Can you work these out from the model? Positions are in its coordinate system, mm. A direction names the side the tool comes from. Round coordinates to 2 decimals unless told otherwise and drop trailing zeros. Loops run counter-clockwise (first coordinate to the right, second up) from the corner with the lowest first, then second, coordinate; pieces in that order, holes last.
from build123d import *

# Parameters (mm, degrees)
CUT_EXTRUDE1_START = 12.7
SKETCH2_R          = 12.7
CUT_EXTRUDE1_DEPTH = 76.2
FILLET2_R          = 15.24


with BuildPart() as part:
    # Sketch1 → Revolve1 (revolve)
    with BuildSketch(Plane.XY, mode=Mode.PRIVATE) as revolve1_sk:
        Polygon((0, 0), (0, 25.4), (50.8, 25.4), (50.8, 152.4), (101.6, 152.4), (101.6, 0), align=None)
    revolve(revolve1_sk.sketch.rotate(Axis((0, 0, 0), (0, 1, 0)), 270), axis=Axis((0, 0, 0), (0, 1, 0)))

    # Sketch2 → Cut-Extrude1 (cut)
    with BuildSketch(Plane.XZ.offset(CUT_EXTRUDE1_START)):
        with Locations(Location((-76.2, 0, 0), (0, 0, 270))):
            Circle(SKETCH2_R)
        with Locations(Location((76.2, 0, 0), (0, 0, 270))):
            Circle(SKETCH2_R)
    extrude(amount=-CUT_EXTRUDE1_DEPTH, mode=Mode.SUBTRACT)

    # Fillet2
    # the kernel refuses this fillet: 15.24 mm, written as the material it takes off along each edge
    with BuildSketch(Plane(origin=(0, 0, 0), x_dir=(0, 0, 1), z_dir=(-1, 0, 0))) as fillet2_piece_1:
        with BuildLine():
            CenterArc((101.6 - FILLET2_R, FILLET2_R), FILLET2_R, 270, 90)
            Line((101.6 - FILLET2_R, 0), (101.6, 0))
            Line((101.6, 0), (101.6, FILLET2_R))
        make_face()
    revolve(axis=Axis((0, 0, 0), (0, 1, 0)), mode=Mode.SUBTRACT)
    with BuildSketch(Plane(origin=(0, 152.4, 0), x_dir=(0, 0, 1), z_dir=(-1, 0, 0))) as fillet2_piece_2:
        with BuildLine():
            CenterArc((101.6 - FILLET2_R, -FILLET2_R), FILLET2_R, 0, 90)
            Line((101.6, -FILLET2_R), (101.6, 0))
            Line((101.6, 0), (101.6 - FILLET2_R, 0))
        make_face()
    revolve(axis=Axis((0, 152.4, 0), (0, 1, 0)), mode=Mode.SUBTRACT)


solid = part.part
(1) If we section it at C-C, the plane y = 72.5: List the corners of the cut face in (x, z) for me.
Worked answers:
outline: circle Ø203.2 at (0, 0); hole circle Ø101.6 at (0, 0)
(2) If we section it at B-B, the plane y = 45: List the corners of the cut face in (x, z) for me, then the cut area to 3 significant figures.
Worked answers:
outline: circle Ø203.2 at (0, 0); hole circle Ø25.4 at (-76.2, 0); hole circle Ø101.6 at (0, 0); hole circle Ø25.4 at (76.2, 0)
area: 23,300 mm2
(3) For faces 1 (the cylindrical face through (63.8, 31.31, 2.75)), 2 (the flat face through (1, 25.4, 1)), 3 (the flat face through (1, 0, -1)), which set-ups out of +Z, -Z, +X, -X, +Y, -Y let a thin tool reach every point of the face, with its end or its side?
Worked answers:
face 1: -Y
face 2: +Y
face 3: +Z, -Z, +X, -X, -Y
(4) If I drill on line 1 (X direction, y = 47.5, z = 0); line 2 (X direction, y = 20, z = 0); line 3 (X direction, y = 94, z = 2.5), over which ranges is the centre line in solid material (lowest first)?
Worked answers:
line 1: x = -101.6 to -88.9, -63.5 to -50.8, 50.8 to 63.5, 88.9 to 101.6
line 2: x = -101.6 to -88.9, -63.5 to 63.5, 88.9 to 101.6
line 3: x = -101.57 to -50.74, 50.74 to 101.57
(5) If we section it at A-A, the plane x = 0: List the corners of the cut face in (y, z) for me.
Worked answers:
outline: (0, -86.36) arc R15.24 ccw to (15.24, -101.6) - (137.16, -101.6) arc R15.24 ccw to (152.4, -86.36) - (152.4, -50.8) - (25.4, -50.8) - (25.4, 50.8) - (152.4, 50.8) - (152.4, 86.36) arc R15.24 ccw to (137.16, 101.6) - (15.24, 101.6) arc R15.24 ccw to (0, 86.36) - close
(6) Will these pins go through, and if not, where does the flat tip stop? P1, Ø6, axis at y = 65, z = -26, coming from the +X side; P2, Ø4, axis at y = 33, z = 8.5, coming from the +X side; P3, Ø5, axis at x = -27, y = 87, coming from the -Z side.
Worked answers:
P1: stops at x = 98.96
P2: stops at x = 101.39
P3: stops at z = -98.6
(7) If we mould it in two halves opening along Z, with no side actions, what happens to faces 4 (the cylindrical face through (-61.82, 75.35, -80.63)), 5 (the cylindrical face through (-30.911, 89.789, -40.313)), 6 (the flat face through (-37, 152.4, -37))? For each: released by +Z, released by -Z, zero draft, split by the parting line, or undercut.
Worked answers:
face 4: split by the parting line
face 5: undercut
face 6: zero draft
